Autodesk Inventor part; units mm, degrees
ref_plane "YZ Plane" through (0, 0, 0) normal (1, 0, 0) x (0, 1, 0)
ref_plane "XZ Plane" through (0, 0, 0) normal (0, 1, 0) x (-1, 0, 0)
ref_plane "XY Plane" through (0, 0, 0) normal (0, 0, 1) x (1, 0, 0)
sketch "Sketch1" plane through (0, 0, 0) normal (1, 0, 0) x (0, 1, 0)
  line L0 (0, 0) -> (1.27, 0)
  line L1 (1.27, 0) -> (1.27, 22.3012)
  line L2 (1.27, 22.3012) -> (0, 22.3012)
  arc A0 (0, 3.7418) -> (-1.4817, 13.594) centre (-15.6464, 6.4262) ccw
  line L3 (0, 18.4404) -> (-1.4817, 13.594)
  line L4 (0, 22.3012) -> (0, 18.4404)
  line L5 (0, 3.7418) -> (0, 0)
  dimension "d0" = 1.27
  dimension "d1" = 22.3012
  dimension "d2" = 31.75
  dimension "d3" = 6.4262
  dimension "d4" = 16.9164
  dimension "d6" = 3.8608
extrude "Extrusion1" add sketch "Sketch1" along normal blind 12.3444
sketch "Sketch2" plane through (0, 1.27, 22.3012) normal (0, 1, 0) x (1, 0, 0)
  line L0 (0, 0) -> (12.3444, 0)
  line L1 (9.9568, 0) -> (9.1694, 3.1581)
  line L2 (11.557, 0) -> (12.3444, 3.1581)
  line L3 (9.1694, 3.1581) -> (9.1694, 19.1431)
  line L4 (12.3444, 22.3012) -> (12.3444, 0)
  line L5 (10.7569, 0) -> (10.7569, 22.3012)
  line L6 (0, 22.3012) -> (12.3444, 22.3012)
  line L7 (9.9568, 22.3012) -> (9.1694, 19.1431)
  line L8 (11.557, 22.3012) -> (12.3444, 19.1431)
  line L9 (9.1694, 19.1431) -> (0, 19.1431)
  line L10 (9.1694, 3.1581) -> (0, 3.1581)
  line L11 (0, 22.3012) -> (0, 0)
  line L12 (0, 19.1431) -> (0, 22.3012)
  line L13 (0, 22.3012) -> (9.9568, 22.3012)
  line L14 (0, 3.1581) -> (0, 0)
  dimension "d9" = 1.6002
  dimension "d13" = 28
  dimension "d14" = 3.175
  dimension "d15" = 1.5875
  dimension "d16" = 1.6002
  dimension "d17" = 28
extrude "Extrusion2" cut sketch "Sketch2" against normal blind 25.4 contours L11 L10 L1 L0 | L11 L6 L7 L9 | L2 L4 L0 | L6 L4 L8
sketch "Sketch8" plane through (0, 1.27, 3.1581) normal (0, 1, 0) x (1, 0, 0)
  line L0 (9.1694, -0.8043) -> (0, -0.8043)
  line L1 (9.1694, 0) -> (0, 0)
  line L2 (0, -0.8043) -> (9.1694, -0.8043)
  line L3 (9.1694, -0.8043) -> (9.1694, 0)
  line L4 (9.1694, 0) -> (0, 0)
  line L5 (0, 0) -> (0, -0.8043)
  point P0 (0, 3.1581)
  point P1 (0, -10.4309)
extrude "Extrusion5" cut sketch "Sketch8" against normal blind 25.4
sketch "Sketch9" plane through (9.9568, 1.27, 22.3012) normal (0, 1, 0) x (1, 0, 0)
  line L0 (-10.6834, 14.9326) -> (-5.2324, 18.3388)
  line L1 (-5.2324, 18.3388) -> (-10.6834, 18.3388)
  line L2 (-10.6834, 18.3388) -> (-10.6834, 14.9326)
  line L3 (-0.7874, 19.1431) -> (-0.7874, 18.3388)
  line L4 (-0.7874, 18.3388) -> (-9.9568, 18.3388)
  point P0 (-9.9568, 22.3012)
  dimension "d41" = 32
  dimension "d42" = 4.445
extrude "Extrusion6" cut sketch "Sketch9" against normal blind 25.4
sketch "Sketch14" plane through (9.9568, 1.27, 22.3012) normal (0, 1, 0) x (1, 0, 0)
  circle A0 centre (-4.5896, 11.2866) radius 1.143
  line L0 (-5.2273, 9.7597) -> (-3.813, 11.1739)
  line L1 (-5.2273, 9.7597) -> (-3.2273, 9.7597) construction
  line L2 (-3.813, 11.1739) -> (-5.2273, 11.1739)
  line L3 (-5.2273, 11.1739) -> (-5.2273, 9.7597)
  line L4 (-3.813, 11.1739) -> (-3.813, 9.7597)
  line L5 (-3.813, 9.7597) -> (-5.2273, 9.7597)
  circle A1 centre (-4.5201, 10.4668) radius 3.175
  point P0 (-9.9568, 22.3012)
  dimension "d78" = 2.286
  dimension "d86" = 2
  dimension "d87" = 45
  dimension "d88" = 6.35
extrude "Extrusion11" cut sketch "Sketch14" against normal blind 25.4 contours A0 L4 L2 L3 | L3 L2 L0 A0 | A0 L0 L4
sketch "Sketch15" plane through (9.9568, 1.27, 22.3012) normal (0, 1, 0) x (1, 0, 0)
  circle A0 centre (-4.5896, 11.2866) radius 1.143
  circle A1 centre (-4.5896, 11.2866) radius 0.9525
  circle A2 centre (-4.5896, 11.2866) radius 4.1275
  point P0 (-9.9568, 22.3012)
  dimension "d82" = 1.905
  dimension "d83" = 8.255
extrude "Extrusion12" cut sketch "Sketch15" against normal blind 2.032 contours A2
sketch "Sketch19" plane through (9.9568, 1.27, 22.3012) normal (0, 1, 0) x (1, 0, 0)
  circle A0 centre (1.0564, 15.0967) radius 0.635
  circle A1 centre (-1.7204, 16.4692) radius 0.635
  circle A2 centre (-4.1782, 17.2168) radius 0.635
  point P0 (-9.9568, 22.3012)
  dimension "d102" = 1.27
  dimension "d103" = 1.27
  dimension "d104" = 1.27
extrude "Extrusion17" cut sketch "Sketch19" against normal blind 2.286
sketch "Sketch27" plane through (9.1694, 0.0362, 3.9624) normal (0, 0, -1) x (-1, 0, 0)
  line L0 (0, 1.2338) -> (0, -0.0362)
  line L1 (9.1694, 1.2338) -> (9.1694, 0.1848)
  line L2 (0, 1.2338) -> (9.1694, 1.2338)
  line L3 (9.1694, 1.2338) -> (9.1694, 0.4718)
  line L4 (9.1694, 0.4718) -> (0, 0.4718)
  line L5 (0, 0.4718) -> (0, 1.2338)
  point P0 (9.1694, -0.0362)
  dimension "d122" = 0.762
extrude "Extrusion22" cut sketch "Sketch27" against normal through all
sketch "Sketch29" plane through (4.7244, 0.508, 3.9624) normal (0, 1, 0) x (1, 0, 0)
  arc A0 (-0.0195, -7.9838) -> (1.3051, -7.9838) centre (0.6428, -7.0522) ccw
  arc A1 (-4.7244, -7.0522) -> (4.445, -10.8404) centre (0.6428, -7.0522) ccw
  line L0 (-4.7244, -15.1807) -> (-4.7244, -2.9521)
  line L1 (4.445, -8.6583) -> (4.445, -15.1807)
  line L2 (4.445, -10.8404) -> (4.445, -15.1807)
  line L3 (4.445, -15.1807) -> (-4.7244, -15.1807)
  point P0 (-4.7244, 3.9624)
extrude "Extrusion23" cut sketch "Sketch29" against normal through all
sketch "Sketch30" plane through (4.7244, 0.508, 3.9624) normal (0, 1, 0) x (1, 0, 0)
  line L0 (0, 0) -> (-4.7244, -2.9521)
  line L1 (-4.7244, -2.9521) -> (-4.7244, -7.0522)
  arc A0 (0, 0) -> (-4.7244, -7.0522) centre (6.8812, -9.7184) ccw
  line L2 (-4.7244, -7.0522) -> (-4.7244, -2.9521)
  point P0 (-4.7244, 3.9624)
extrude "Extrusion24" cut sketch "Sketch30" against normal through all
sketch "Sketch32" plane through (9.1694, 0.0362, 3.9624) normal (0, 0, -1) x (-1, 0, 0)
  line L0 (4.445, 0.4718) -> (0, 0.4718)
  line L1 (0, 0.4718) -> (0, 1.2338)
  line L2 (0, 1.2338) -> (-3.175, 1.2338)
  line L3 (0, 0.4718) -> (0, 0)
  line L4 (-3.175, 1.2338) -> (0, 0.4718)
  point P0 (9.1694, -0.0362)
extrude "Extrusion26" cut sketch "Sketch32" against normal blind 12.7
sketch "Sketch37" plane through (4.7244, 0.508, 3.9624) normal (0, 1, 0) x (1, 0, 0)
  arc A0 (4.445, -5.4461) -> (4.445, -8.6583) centre (0.6428, -7.0522) ccw
  arc A1 (4.445, -1.4721) -> (-0.5374, -0.4038) centre (0.6428, -7.0522) ccw
  line L0 (4.445, 0) -> (4.445, -5.4461)
  line L1 (4.445, -1.4721) -> (4.445, 0)
  line L2 (4.445, 0) -> (0, 0)
  arc A2 (0, 0) -> (-4.7244, -7.0522) centre (6.8812, -9.7184) ccw
  line L3 (0, 0) -> (4.445, 0)
  arc A3 (0, 0) -> (-0.5374, -0.4038) centre (1.2434, -2.2145) ccw
  point P0 (-4.7244, 3.9624)
extrude "Extrusion27" cut sketch "Sketch37" against normal blind 12.7 contours A1 A2 L2 L0
chamfer "Chamfer4" distance 0.762 angle 45 1 edges at (1.2397, 0.508, 11.0146)
sketch "Sketch38" plane through (9.9568, -0.762, 22.3012) normal (0, 1, 0) x (1, 0, 0)
  ellipse E0 centre (-3.5768, 11.2866) end of major axis (-7.7968, 11.2866) minor radius 4.0967 (-3.9624, 7.207) -> (-0.7874, 8.2124) ccw
  arc A0 (-4.2943, 7.198) -> (-4.2943, 15.3752) centre (-3.5768, 11.2866) ccw
  arc A1 (-3.9624, 7.207) -> (-2.158, 14.6218) centre (-4.5896, 11.2866) ccw
  arc A2 (-4.2943, 7.198) -> (-4.2943, 15.3752) centre (-4.5896, 11.2866) ccw
  point P0 (-9.9568, 22.3012)
extrude "Extrusion28" cut sketch "Sketch38" along normal blind 12.7
sketch "Sketch39" plane through (5.3672, 0.508, 11.0146) normal (0, 1, 0) x (1, 0, 0)
  point P0 (-5.3672, 11.0146)
equation "\"d15\" = 0.5 * d14"
properties part number "headppost_Turi_2gen"
The listing builds one solid part. Answer for the finished solid, in the listing's coordinates (mm). A direction names the side the tool comes from. Coordinates: 2 decimals unless noted, no trailing zeros. Write each loop counter-clockwise with the first axis right and the second up, starting at its lowest first coordinate (ties: lowest second). Pieces come first, ordered by that corner, then holes. Notation, with made-up numbers: (66, 22) - (94, 22) arc R13 cw to (94, 26) - close; hole circle Ø4 at (59.25, 70.5). An arc over 180 degrees is marked (long way). Return JSON: item names as keys, results as strings. Group by question number.
1. A cutting plane is placed at B-B, the plane z = 7.5. Give the number of separate pieces and of enclosed holes in the cut face, plus the area to 3 significant figures.
2. A cutting plane is placed at D-D, the plane z = 19.5. Determine the outline of the cut face in (x, y), plus the area to 3 significant figures.
3. Which of the six approach directions +Z, -Z, +X, -X, +Y, -Y give full straight-line access (tool end or side, diameter ignored) to faces 5 (the cylindrical face through (9.913, 0.026, 13.193)), 6 (the cylindrical face through (1.11, 0.355, 8.055)), 7 (the flat face through (6, -0.762, 13)), 8 (the flat face through (9.169, 0, 17))?
4. Given pin 1 (0.7 mm diameter, centred on y = 0.5, z = 17.5, fed in from -X); pin 2 (1.4 mm diameter, centred on y = 0.5, z = 4, fed in from -X); pin 3 (1 mm diameter, centred on x = 3, y = -0.5, fed in from +Z); pin 4 (6 mm diameter, centred on x = 4, z = 15.5, fed in from -Y), each flat-ended and moving along its own axis, determine where each tip first touches the part or whether it passes through.
5. Determine the mould class of faces 1 (the conical face through (1.65, -0.12, 13.1)), 2 (the flat face through (11, 0, 2)), 3 (the cylindrical face through (11.6, 0.54, 7.45)), 4 (the cylindrical face through (3.236, -0.252, 15.941)) for opening direction Z: released by +Z, released by -Z, zero draft, split by the parting line, or undercut.
6. Straight lines are drawn through the part: L1, parallel to Y at x = 9.25, z = 3; L2, parallel to Z at x = 10.75, y = 1; L3, parallel to X at y = -0.05, z = 18. For each, find the intervals that lie inside material, in ascending order.
7. A cutting plane is placed at A-A, the plane x = 9.5. Determine the outline of the cut face in (y, z).
Ans:
{
 "1": {"separate pieces": "3", "enclosed holes": "0", "area": "1.78 mm²"},
 "2": {"outline": "(9.26, 0) - (12.26, 0) - (12.26, 1.27) - (9.26, 1.27) - close", "area": "3.81 mm²"},
 "3": {"face 5": "+Y", "face 6": "-Z, -X, +Y, -Y", "face 7": "-Z, +Y", "face 8": "+Z, +Y, -Y"},
 "4": {"pin 1": "x = 9.17", "pin 2": "x = 3.79", "pin 3": "z = 16.05", "pin 4": "y = -1.48"},
 "5": {"face 1": "undercut", "face 2": "zero draft", "face 3": "undercut", "face 4": "released by +Z"},
 "6": {"L1": "0 to 1.27", "L2": "0 to 3.96, 16.66 to 22.3", "L3": "9.17 to 12.34"},
 "7": {"outline": "(-1.48, 13.59) arc R15.88 cw to (-0.76, 11.95) - (-0.76, 13.75) - (0.59, 13.75) - (0.59, 16.66) - (1.27, 16.66) - (1.27, 20.47) - (0, 20.47) - (0, 18.44) - close; (0, 1.83) - (1.27, 1.83) - (1.27, 3.96) - (0.59, 3.96) - (0.59, 8.28) - (0.12, 8.28) arc R15.88 cw to (0, 3.74) - close"}
}
